Study the drawing (mm; zero at the part's minimum x, y, z) and answer. A direction names the side the tool comes from. Coordinates: 2 decimals unless noted, no trailing zeros. Answer in a Markdown table with one row per item. Add a question column.
Item 1: For a pull along Y with two mould halves and no side action, classify the marked faces 1, 2 and 3 as +Y half, -Y half, draft (parallel to the pull), parting line (faces both ways), or undercut.
Item 2: Given pin 1 Ø9.5 at (x, z) = (85.5, 10.5) entering from +Y (3 decimals); pin 2 Ø9.5 at (x, z) = (89.5, 7.5) entering from -Y; pin 3 Ø9.5 at (y, z) = (8, 8) entering from +X (3 decimals), each flat-ended and moving along its own axis, determine where each tip first touches the part or whether it passes through.
Item 3: Which of the six approach directions +Z, -Z, +X, -X, +Y, -Y give full straight-line access (tool end or side, diameter ignored) to the marked faces 4, 5, 6 and 7?
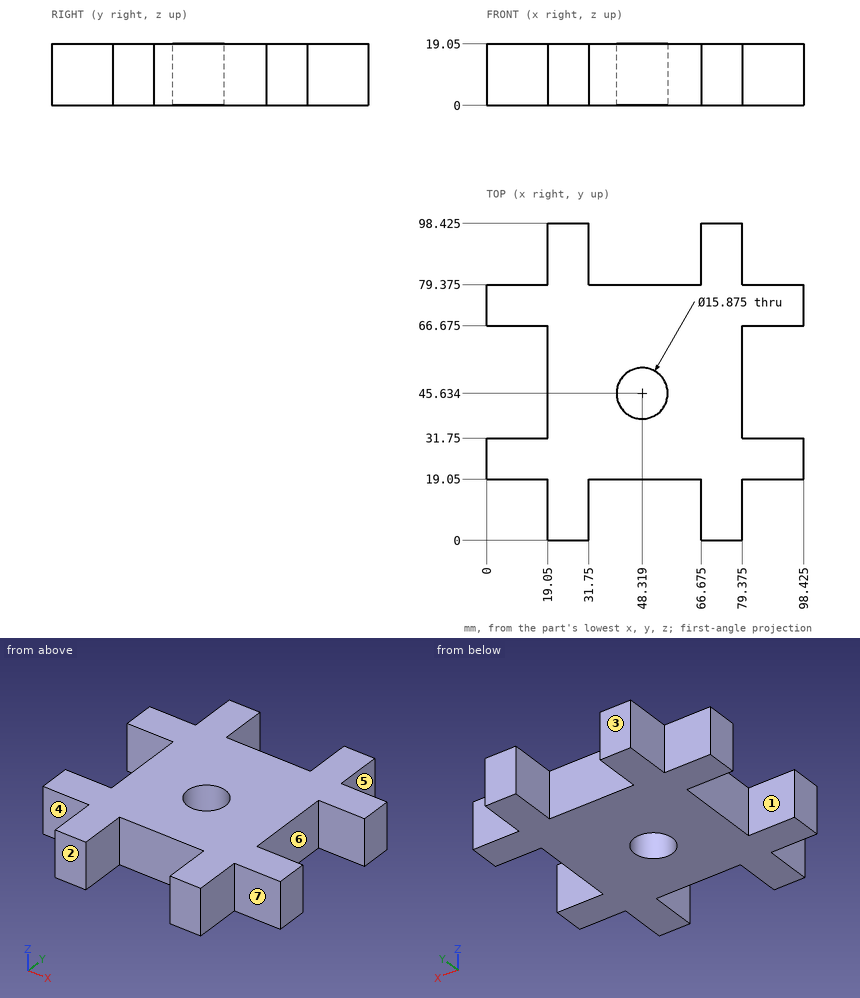
Results below:
| question | item | result |
|---|---|---|
| 1 | face 1 | undercut |
| 1 | face 2 | -Y half |
| 1 | face 3 | +Y half |
| 2 | pin 1 | stops at y = 79.375 |
| 2 | pin 2 | stops at y = 19.05 |
| 2 | pin 3 | stops at x = 79.375 |
| 3 | face 4 | +Z, -Z, -X, -Y |
| 3 | face 5 | +Z, -Z, +X, +Y |
| 3 | face 6 | +Z, -Z, +X |
| 3 | face 7 | +Z, -Z, +X, -Y |
